Source: CAD feature listing. Evaluate the final solid. Frame: model axes, mm. Give positions to 0.01 mm unless a question says otherwise; leave off trailing zeros. Loops run counter-clockwise (first coordinate to the right, second up) from the corner with the lowest first, then second, coordinate; pieces in that order, holes last. Notation, with made-up numbers: M 65.25,50.25 L 70.25,50.25 A30 ccw 70.25,75.25 Z; hole C -10.75,-2 d1. An arc over 180 degrees is marked long. Answer in a Markdown table with one row per item.
```python
from build123d import *

# Parameters (mm, degrees)
SKETCH_1_W          = 20
SKETCH_1_H          = 48
EXTRUDE_1_DEPTH     = 3
SKETCH_2_R          = 1.525
CUT_EXTRUDE_1_DEPTH = 4
FILLET_1_R          = 2


with BuildPart() as part:
    # 草图1 → 凸台-拉伸1 (new body)
    with BuildSketch(Plane(origin=(0, 0, 0), x_dir=(1, 0, 0), z_dir=(0, 1, 0))):
        Rectangle(SKETCH_1_W, SKETCH_1_H)
    extrude(amount=EXTRUDE_1_DEPTH)

    # 草图2 → 切除-拉伸1 (cut, through all)
    with BuildSketch(Plane(origin=(0, 3, 0), x_dir=(1, 0, 0), z_dir=(0, 1, 0))):
        with Locations((7, 0)):
            Circle(SKETCH_2_R)
        with Locations((7, 20)):
            Circle(SKETCH_2_R)
        with Locations((-4, 0)):
            Circle(SKETCH_2_R)
        with Locations((-4, 15)):
            Circle(SKETCH_2_R)
        with Locations((7, -20)):
            Circle(SKETCH_2_R)
        with Locations((-4, -15)):
            Circle(SKETCH_2_R)
    extrude(amount=-CUT_EXTRUDE_1_DEPTH, mode=Mode.SUBTRACT)

    # 圆角1
    fillet_1_edges = [part.edges().sort_by_distance(p)[0] for p in [
        (10, 1.5, 24),
        (-10, 1.5, 24),
        (-10, 1.5, -24),
        (10, 1.5, -24),
    ]]
    fillet(fillet_1_edges, radius=FILLET_1_R)


solid = part.part
```
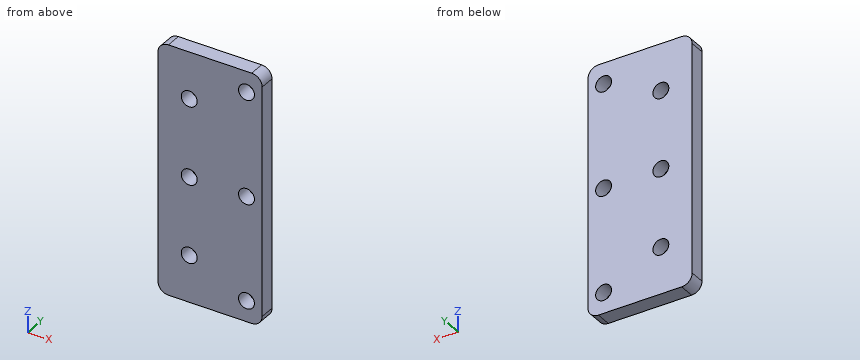
Q1. Section query A-A (x = 7). Output: boundary loops of the cut face in (y, z) (3 decimals).
Values follow:
| item | result |
|---|---|
| outline | M 0,-24 L 3,-24 L 3,-21.525 L 0,-21.525 Z; M 0,-18.475 L 3,-18.475 L 3,-1.525 L 0,-1.525 Z; M 0,1.525 L 3,1.525 L 3,18.475 L 0,18.475 Z; M 0,21.525 L 3,21.525 L 3,24 L 0,24 Z |
Q2. Section query C-C (y = 1.25). Output: boundary loops of the cut face in (x, z) (3 decimals).
Values follow:
| item | result |
|---|---|
| outline | M -10,-22 A2 ccw -8,-24 L 8,-24 A2 ccw 10,-22 L 10,22 A2 ccw 8,24 L -8,24 A2 ccw -10,22 Z; hole C -4,-15 d3.05; hole C -4,0 d3.05; hole C -4,15 d3.05; hole C 7,-20 d3.05; hole C 7,0 d3.05; hole C 7,20 d3.05 |
Q3. Section query D-D (z = -0.5). Output: boundary loops of the cut face in (x, y), plus the area to 3 significant figures.
Values follow:
| item | result |
|---|---|
| outline | M -10,0 L -5.44,0 L -5.44,3 L -10,3 Z; M -2.56,0 L 5.56,0 L 5.56,3 L -2.56,3 Z; M 8.44,0 L 10,0 L 10,3 L 8.44,3 Z |
| area | 42.7 mm^2 |
Q4. Contact query for a flat-ended pin moving along its axis: pin 1 Ø1.8 at (x, z) = (7, 20) entering from -Y. Output: stop coordinate, or through.
Values follow:
| item | result |
|---|---|
| pin 1 | through |
Q5. Ray query, probe 1 along Z at (x, y) = (-4, 1.2) (3 decimals); probe 2 along Z at (x, y) = (7, 1.05) (3 decimals); probe 3 along X at (y, z) = (1.5, 0) (3 decimals). Return the intervals inside material, ascending. Write a range as from..to.
Values follow:
| item | result |
|---|---|
| probe 1 | -24..-16.525, -13.475..-1.525, 1.525..13.475, 16.525..24 |
| probe 2 | -24..-21.525, -18.475..-1.525, 1.525..18.475, 21.525..24 |
| probe 3 | -10..-5.525, -2.475..5.475, 8.525..10 |
Q6. Section query B-B (z = -15). Output: boundary loops of the cut face in (x, y) (3 decimals), plus the area to 4 significant figures.
Values follow:
| item | result |
|---|---|
| outline | M -10,0 L -5.525,0 L -5.525,3 L -10,3 Z; M -2.475,0 L 10,0 L 10,3 L -2.475,3 Z |
| area | 50.85 mm^2 |
